The drawing under review shows one solid part. Ordinate dimensions are in mm from its lowest x, y, z. A direction names the side the tool comes from. Give positions to 0.01 mm unless a question says otherwise; leave off trailing zeros. Loops run counter-clockwise (first coordinate to the right, second up) from the corner with the lowest first, then second, coordinate; pieces in that order, holes last. Notation, with made-up numbers: M -29,81.25 L -23,81.25 A12 cw -23,90.25 Z; hole C -22,-21.75 d10. An arc over 180 degrees is marked long. Put each result on its own line as item: value. Start each with the question number.
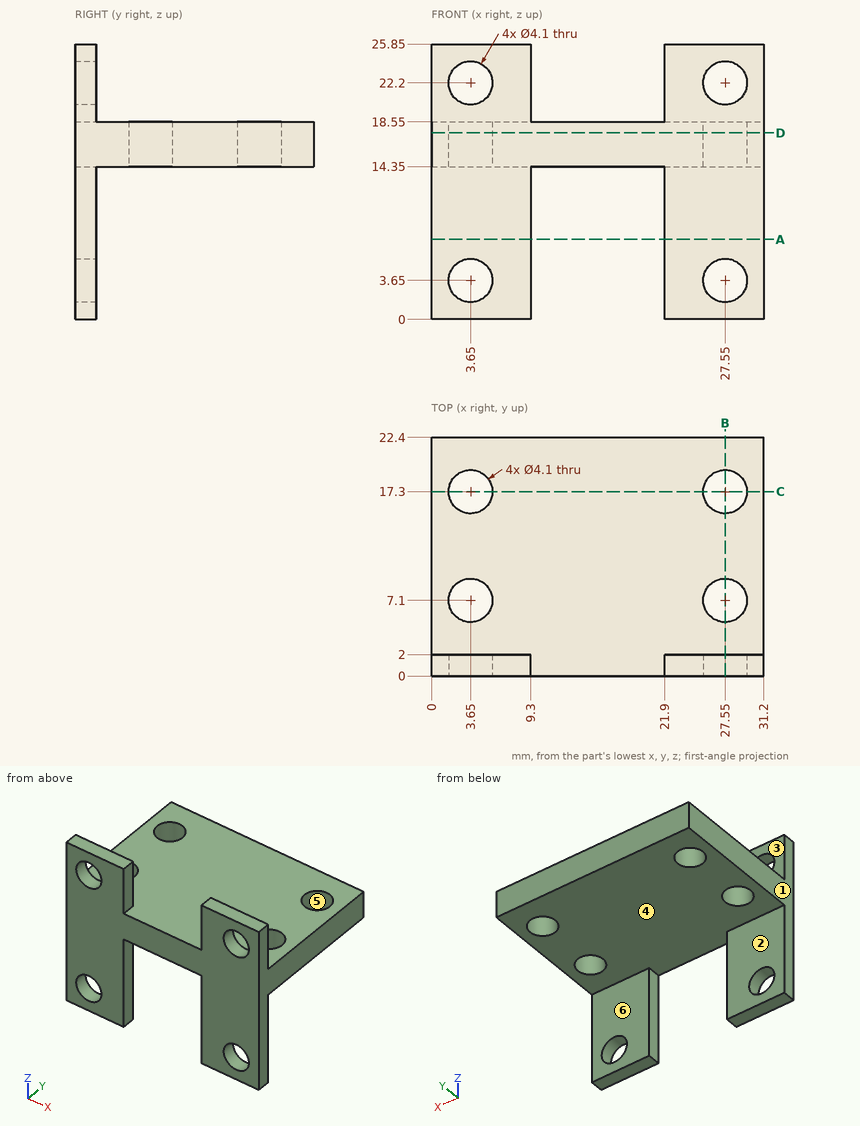
Item 1: Consider section B-B, the plane x = 27.55. Write out the cut boundary in (y, z), plus the area to 3 significant figures.
Item 2: Draft analysis for pull direction Y (two halves, no side actions). For the marked faces 4, 5 and 6, state which applies: +Y half, -Y half, draft (parallel to the pull), parting line (faces both ways), or undercut.
Item 3: Consider section D-D, the plane z = 17.5. Write out the cut boundary in (x, y), plus the area to 3 significant figures.
Item 4: Tool access review of the marked faces 1, 2 and 3: name each direction out of +Z, -Z, +X, -X, +Y, -Y from which nothing blocks a thin tool from reaching the whole face with its end or side.
Item 5: Consider section C-C, the plane y = 17.3. Write out the cut boundary in (x, z).
Item 6: Consider section A-A, the plane z = 7.5. Write out the cut boundary in (x, y).
Item 7: To check wall thickness, follow L1, parallel to Y at x = 3.65, z = 16.6; L2, parallel to X at y = 0.6, z = 3.65; L3, parallel to Z at x = 30, y = 21. State the ranges of each line that lie inside material, in increasing order. Write a range as [from, to].
Item 8: Clearance check with flat-ended pins moving along their axes: pin 1 Ø2 at (x, z) = (6.5, 6) entering from +Y; pin 2 Ø3.5 at (x, y) = (27.55, 7.1) entering from +Z; pin 3 Ø11 at (x, y) = (14.5, 12.5) entering from -Z. State where each tip first meets the part, or that it passes through.
Report:
1. outline: M 0,0 L 2,0 L 2,1.6 L 0,1.6 Z; M 0,5.7 L 2,5.7 L 2,14.35 L 5.05,14.35 L 5.05,18.55 L 2,18.55 L 2,20.15 L 0,20.15 Z; M 0,24.25 L 2,24.25 L 2,25.85 L 0,25.85 Z; M 9.15,14.35 L 15.25,14.35 L 15.25,18.55 L 9.15,18.55 Z; M 19.35,14.35 L 22.4,14.35 L 22.4,18.55 L 19.35,18.55 Z
1. area: 86.5 mm²
2. face 4: draft
2. face 5: undercut
2. face 6: +Y half
3. outline: M 0,0 L 31.2,0 L 31.2,22.4 L 0,22.4 Z; hole C 3.65,7.1 d4.1; hole C 3.65,17.3 d4.1; hole C 27.55,7.1 d4.1; hole C 27.55,17.3 d4.1
3. area: 646 mm²
4. face 1: +Z, -Z, -X, +Y, -Y
4. face 2: -Z, +X, -X, +Y
4. face 3: +Z, +X, -X, +Y
5. outline: M 0,14.35 L 1.6,14.35 L 1.6,18.55 L 0,18.55 Z; M 5.7,14.35 L 25.5,14.35 L 25.5,18.55 L 5.7,18.55 Z; M 29.6,14.35 L 31.2,14.35 L 31.2,18.55 L 29.6,18.55 Z
6. outline: M 0,0 L 9.3,0 L 9.3,2 L 0,2 Z; M 21.9,0 L 31.2,0 L 31.2,2 L 21.9,2 Z
7. L1: [0, 5.05], [9.15, 15.25], [19.35, 22.4]
7. L2: [0, 1.6], [5.7, 9.3], [21.9, 25.5], [29.6, 31.2]
7. L3: [14.35, 18.55]
8. pin 1: y = 2
8. pin 2: through
8. pin 3: z = 14.35
